Build history of the part. All positions in model axes, mm. A direction names the side the tool comes from. Round coordinates to 2 decimals unless told otherwise and drop trailing zeros. Order: outer loops, then holes, each group sorted by start corner. A loop starts at its lowest first (then second) coordinate and runs counter-clockwise, first axis right, second up. Notation, with made-up numbers: (-9.75, 22.5) -> (5.25, 22.5) arc R7 ccw to (5.25, 27.5) -> close; hole circle Ø2 at (10, 64.25). An arc over 180 degrees is marked (long way). Use a Markdown table: item, result. Add a question column.
Item 1: Two-plate mould, pull along Z, no slides. Class faces 1 (the face through (8.315, -19.699, 10.215)), 2 (the face through (8.315, -19.715, -10.199)), 3 (the face through (18, 25, -3.2)): released by +Z, released by -Z, zero draft, split by the parting line, or undercut.
Item 2: Slice it at A-A, the plane z = 5.2. Give the cut face in (x, y), plus the area to 3 significant figures.
Item 3: Slice it at C-C, the plane y = 12. Give the cut face in (x, z).
Item 4: Pin check, flat tips, straight feed: pin 1 (10.5 mm diameter, centred on y = -6, z = -4.5, fed in from +X); pin 2 (5 mm diameter, centred on x = 24, z = -1, fed in from -Y); pin 3 (1.5 mm diameter, centred on x = 9.5, y = 20, fed in from -Z). Stop position of each tip, or through.
Item 5: Slice it at D-D, the plane z = 8. Give the cut face in (x, y).
Item 6: Probe L1, parallel to Y at x = 21.5, z = -8.25; L2, parallel to X at y = 4, z = -7.5; L3, parallel to X at y = 21, z = 9. List the from-to ranges inside material, lowest first.
Item 7: Slice it at B-B, the plane x = 8. Give the cut face in (y, z).
Item 8: 3-axis set-ups, long thin cutter, end or side, ignore diameter. For faces 4 (the face through (19.4, -23, 0)), 5 (the face through (18, 26, -7.2)), 6 (the face through (18, -26, -7.2)), 7 (the face through (19.4, 23, 0)), 8 (the face through (8.315, 19.715, -10.199)): which of +Z, -Z, +X, -X, +Y, -Y reach the whole face in a straight line?
from build123d import *

# Parameters (mm, degrees)
SKETCH1_W            = 21
SKETCH1_H            = 40
BOSS_EXTRUDE1_DEPTH  = 16.4
SKETCH2_W            = 21
SKETCH2_H            = 54
BOSS_EXTRUDE2_DEPTH  = 3
CUT_EXTRUDE1_DEPTH   = 3
MIRROR2_COPY_1_DEPTH = 3
SKETCH5_W            = 21
SKETCH5_H            = 40
BOSS_EXTRUDE4_DEPTH  = 6
SKETCH6_R            = 3
BOSS_EXTRUDE5_DEPTH  = 0.01
FILLET1_R            = 1
SKETCH9_R            = 3
BOSS_EXTRUDE7_DEPTH  = 3.9878


with BuildPart() as part:
    # Sketch1 → Boss-Extrude1 (new body)
    with BuildSketch(Plane(origin=(0, 0, 0), x_dir=(0, 0, -1), z_dir=(1, 0, 0))):
        Rectangle(SKETCH1_W, SKETCH1_H)
    extrude(amount=BOSS_EXTRUDE1_DEPTH)

    # Sketch2 → Boss-Extrude2 (add)
    with BuildSketch(Plane(origin=(16.4, 0, 0), x_dir=(0, 0, -1), z_dir=(1, 0, 0))):
        Rectangle(SKETCH2_W, SKETCH2_H)
    extrude(amount=BOSS_EXTRUDE2_DEPTH)

    # Sketch3 → Cut-Extrude1 (cut)
    with BuildSketch(Plane(origin=(19.4, 0, 0), x_dir=(0, 0, -1), z_dir=(1, 0, 0))):
        with BuildLine():
            Line((-3.200000014, 24), (-3.200000014, 27))
            Line((-3.200000014, 27), (-7.200000014, 27))
            Line((-7.200000014, 27), (-7.200000014, 24))
            ThreePointArc((-7.200000014, 24), (-5.200000014, 22), (-3.200000014, 24))
        make_face()
    cut_extrude1 = extrude(amount=-CUT_EXTRUDE1_DEPTH, mode=Mode.SUBTRACT)

    # Mirror1: Cut-Extrude1 across plane
    add(cut_extrude1.mirror(Plane.XY), mode=Mode.SUBTRACT)

    # Mirror2: Cut-Extrude1 across plane
    add(cut_extrude1.mirror(Plane.ZX), mode=Mode.SUBTRACT)

    # Mirror2 copy 1 sketch → Mirror2 copy 1 (cut)
    with BuildSketch(Plane(origin=(19.4, 0, 0), x_dir=(0, 0, 1), z_dir=(1, 0, 0))):
        with BuildLine():
            Line((-3.200000014, 24), (-3.200000014, 27))
            Line((-3.200000014, 27), (-7.200000014, 27))
            Line((-7.200000014, 27), (-7.200000014, 24))
            ThreePointArc((-7.200000014, 24), (-5.200000014, 22), (-3.200000014, 24))
        make_face()
    extrude(amount=-MIRROR2_COPY_1_DEPTH, mode=Mode.SUBTRACT)

    # Sketch5 → Boss-Extrude4 (add)
    with BuildSketch(Plane(origin=(19.4, 0, 0), x_dir=(0, 0, -1), z_dir=(1, 0, 0))):
        Rectangle(SKETCH5_W, SKETCH5_H)
    extrude(amount=BOSS_EXTRUDE4_DEPTH)

    # Sketch6 → Boss-Extrude5 (add)
    with BuildSketch(Plane(origin=(25.4, 0, 0), x_dir=(0, 0, -1), z_dir=(1, 0, 0))):
        with Locations((0, 11.4)):
            Circle(SKETCH6_R)
    extrude(amount=BOSS_EXTRUDE5_DEPTH)

    # Fillet1
    fillet1_edges = [part.edges().sort_by_distance(p)[0] for p in [
        (8.2, -20, -10.5),
        (8.2, -20, 10.5),
        (8.2, 20, 10.5),
        (8.2, 20, -10.5),
    ]]
    fillet(fillet1_edges, radius=FILLET1_R)

    # Sketch9 → Boss-Extrude7 (add)
    with BuildSketch(Plane(origin=(25.41, 0, 0), x_dir=(0, 0, -1), z_dir=(1, 0, 0))):
        with Locations((0, 11.4)):
            Circle(SKETCH9_R)
    extrude(amount=BOSS_EXTRUDE7_DEPTH)


solid = part.part
Check sheet entries:
| question | item | result |
|---|---|---|
| 1 | face 1 | released by +Z |
| 1 | face 2 | released by -Z |
| 1 | face 3 | undercut |
| 2 | outline | (0, -20) -> (16.4, -20) -> (16.4, -22) -> (19.4, -22) -> (19.4, -20) -> (25.4, -20) -> (25.4, 20) -> (19.4, 20) -> (19.4, 22) -> (16.4, 22) -> (16.4, 20) -> (0, 20) -> close |
| 2 | area | 1,030 mm2 |
| 3 | outline | (0, -10.5) -> (25.4, -10.5) -> (25.4, -2.94) -> (29.4, -2.94) -> (29.4, 2.94) -> (25.4, 2.94) -> (25.4, 10.5) -> (0, 10.5) -> close |
| 4 | pin 1 | x = 25.4 |
| 4 | pin 2 | y = -20 |
| 4 | pin 3 | z = -10.47 |
| 5 | outline | (0, -20) -> (16.4, -20) -> (16.4, -27) -> (19.4, -27) -> (19.4, -20) -> (25.4, -20) -> (25.4, 20) -> (19.4, 20) -> (19.4, 27) -> (16.4, 27) -> (16.4, 20) -> (0, 20) -> close |
| 6 | L1 | -20 to 20 |
| 6 | L2 | 0 to 25.4 |
| 6 | L3 | 16.4 to 19.4 |
| 7 | outline | (-20, -9.5) arc R1 ccw to (-19, -10.5) -> (19, -10.5) arc R1 ccw to (20, -9.5) -> (20, 9.5) arc R1 ccw to (19, 10.5) -> (-19, 10.5) arc R1 ccw to (-20, 9.5) -> close |
| 8 | face 4 | +Z, -Z, +X, -Y |
| 8 | face 5 | +X, -X, +Y |
| 8 | face 6 | +X, -X, -Y |
| 8 | face 7 | +Z, -Z, +X, +Y |
| 8 | face 8 | -Z, -X, +Y |
